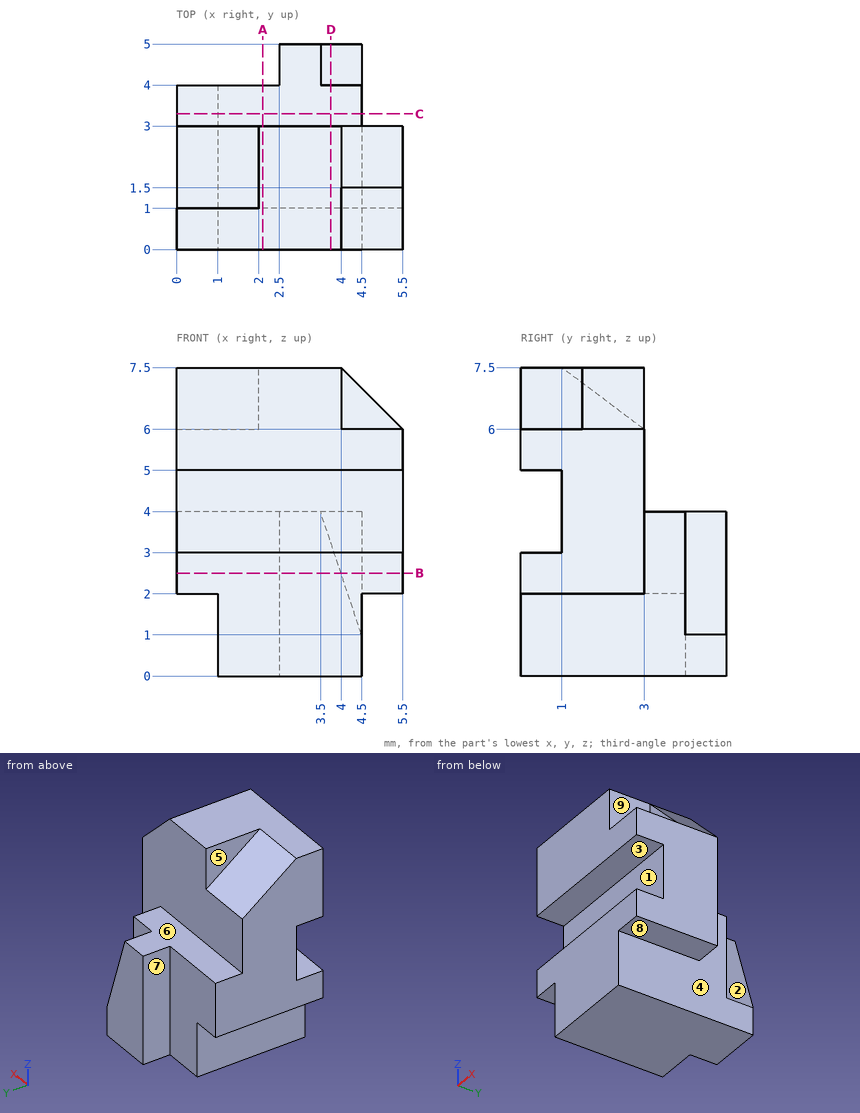
The figure shows three views and two pictorial views of one solid part (mm, origin at its lowest corner). Answer the questions. A direction names the side the tool comes from. Coordinates: 2 decimals unless noted, no trailing zeros. Loops run counter-clockwise (first coordinate to the right, second up) from the corner with the lowest first, then second, coordinate; pieces in that order, holes last. Notation, with made-up numbers: (-32.5, 53.5) -> (-28.5, 53.5) arc R27 cw to (-28.5, 86.5) -> close; hole circle Ø11 at (-6.75, -1.5). An arc over 180 degrees is marked (long way). Write item = value, one per line. Start each with the question number.
1) A cutting plane is placed at C-C (y = 3.3). Give the vertices of the cut face in (x, z), then the cut area to 3 significant figures.
2) A cutting plane is placed at D-D (x = 3.75). Give the vertices of the cut face in (y, z).
3) The mould has two halves that part along Z. Classify the marked faces 1, 2, 3 and 4: released by +Z, released by -Z, zero draft, split by the parting line, or undercut.
4) A cutting plane is placed at A-A (x = 2.1). Give the vertices of the cut face in (y, z).
5) Straight lines are drawn through the part: line 1 (Z direction, x = 5.2, y = 0.45); line 2 (Z direction, x = 3.45, y = 0.2); line 3 (Y direction, x = 2.1, z = 6). For each, find the intervals that lie inside material, in ascending order. Write a range as from..to.
6) A tool of negligible diameter and unlimited length cuts with its end or side. For the marked faces 5, 6, 7, 8 and 9, from which of +Z, -Z, +X, -X, +Y, -Y can it reach the whole face along a straight path? Write none if from no direction.
7) A cutting plane is placed at B-B (z = 2.5). Give the vertices of the cut face in (x, y), then the cut area to 3 significant figures.
8) Given pin 1 Ø1 at (x, y) = (1, 3) entering from +Z (3 decimals); pin 2 Ø1.2 at (x, z) = (5, 6.5) entering from -Y; pin 3 Ø1.6 at (y, z) = (3, 1) entering from -X; pin 4 Ø1.6 at (x, y) = (3, 4) entering from +Z, each flat-ended and moving along its own axis, determine where each tip first touches the part or whether it passes through.
Responses:
q1.outline = (0, 2) -> (1, 2) -> (1, 0) -> (4.5, 0) -> (4.5, 4) -> (0, 4) -> close
q1.area = 16.0 mm²
q2.outline = (0, 0) -> (5, 0) -> (5, 3.25) -> (4, 3.25) -> (4, 4) -> (3, 4) -> (3, 7.5) -> (0, 7.5) -> (0, 5) -> (1, 5) -> (1, 3) -> (0, 3) -> close
q3.face_1 = undercut
q3.face_2 = released by +Z
q3.face_3 = undercut
q3.face_4 = zero draft
q4.outline = (0, 0) -> (4, 0) -> (4, 4) -> (3, 4) -> (3, 7.5) -> (0, 7.5) -> (0, 5) -> (1, 5) -> (1, 3) -> (0, 3) -> close
q5.line_1 = 2..3, 5..6
q5.line_2 = 0..3, 5..7.5
q5.line_3 = 0..3
q6.face_5 = +Z, -X, +Y
q6.face_6 = +Z, +X, -X, +Y
q6.face_7 = +Z, -Z, -X, +Y
q6.face_8 = -Z, +X, +Y, -Y
q6.face_9 = +Z, +X, -Y
q7.outline = (0, 0) -> (5.5, 0) -> (5.5, 3) -> (4.5, 3) -> (4.5, 4) -> (4, 4) -> (4, 5) -> (2.5, 5) -> (2.5, 4) -> (0, 4) -> close
q7.area = 22.5 mm²
q8.pin_1 = 6.375
q8.pin_2 = 0
q8.pin_3 = 1
q8.pin_4 = 4
